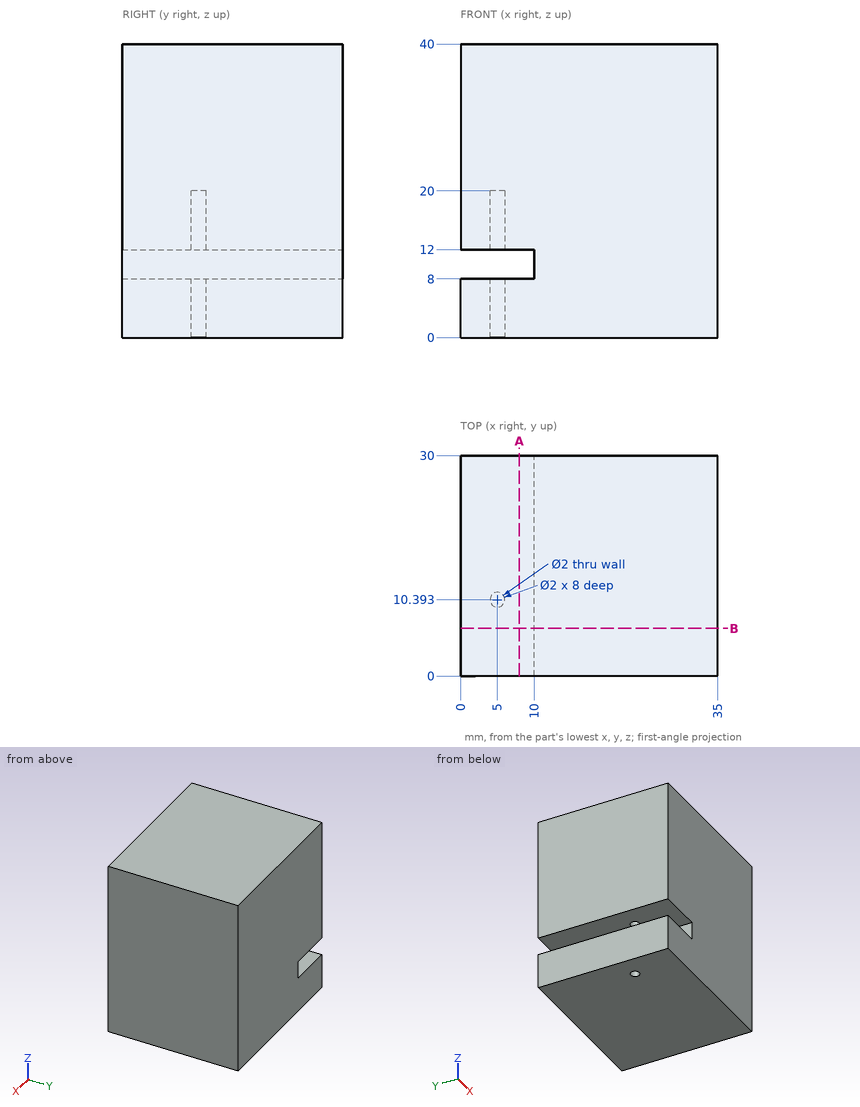
Could you check a few things on this drawing? It's one solid part, dimensions in mm from its lowest x, y, z. Coordinates: 2 decimals unless noted, no trailing zeros. Write each loop counter-clockwise with the first axis right and the second up, starting at its lowest first coordinate (ties: lowest second). Pieces come first, ordered by that corner, then holes.
1) I'm going to push flat-ended pins straight in: pin 1 (1.8 mm diameter, centred on x = 5, y = 10.39, fed in from -Z); pin 2 (1.2 mm diameter, centred on y = 10, z = 10.5, fed in from -X). Where does each tip first touch, or does it pass through?
Filled in:
pin 1: stops at z = 20
pin 2: stops at x = 10
2) If I drill on line 1 (Y direction, x = 5, z = 5.5); line 2 (Z direction, x = 1, y = 28.5); line 3 (X direction, y = 2, z = 11), over which ranges is the centre line in solid material (lowest first)?
Filled in:
line 1: y = 0 to 9.39, 11.39 to 30
line 2: z = 0 to 8, 12 to 40
line 3: x = 10 to 35
3) If we section it at B-B (y = 6.5): List the corners of the cut face in (x, z) for me.
Filled in:
outline: (0, 0) - (35, 0) - (35, 40) - (0, 40) - (0, 12) - (10, 12) - (10, 8) - (0, 8) - close
4) If we section it at A-A (x = 8): List the corners of the cut face in (y, z) for me, plus the area to 3 significant figures.
Filled in:
outline: (0, 0) - (30, 0) - (30, 8) - (0, 8) - close; (0, 12) - (30, 12) - (30, 40) - (0, 40) - close
area: 1,080 mm2
